Print and shaded views of the part. All mm, measured from the part's lowest x, y and z. Coordinates: 2 decimals unless noted, no trailing zeros. Order: outer loops, then holes, each group sorted by start corner. A loop starts at its lowest first (then second) coordinate and runs counter-clockwise, first axis right, second up. Notation, with made-up numbers: (-38, 75.25) -> (-1, 75.25) arc R21 cw to (-1, 89.25) -> close; hole circle Ø3 at (31, -3). An arc over 180 degrees is marked (long way). Return JSON: item names as keys, results as strings. Group by question number.
1) Cut at A-A (z = 43). Write the cut outline in (x, y), and give its area (3 significant figures).
2) Flat gauge pins, fed straight in: pin 1 (4.5 mm diameter, centred on x = 96.5, y = 6.5, fed in from -Z); pin 2 (4.5 mm diameter, centred on x = 80, y = 6, fed in from +Z); pin 3 (1 mm diameter, centred on y = 4, z = 59.5, fed in from +X). Where does each tip first touch, or does it go through?
3) Cut at C-C (z = 27.5). Write the cut outline in (x, y), and give its area (3 significant figures).
4) Cut at B-B (x = 50). Write the cut outline in (y, z), and give its area (3 significant figures).
5) Probe line 1 (X direction, y = 3.25, z = 58.5); line 2 (X direction, y = 3.5, z = 27.5); line 3 (Z direction, x = 65.5, y = 6). List the from-to ranges inside material, lowest first.
6) Cut at D-D (y = 6). State how many separate pieces and enclosed holes the cut face has, and give its area (3 significant figures).
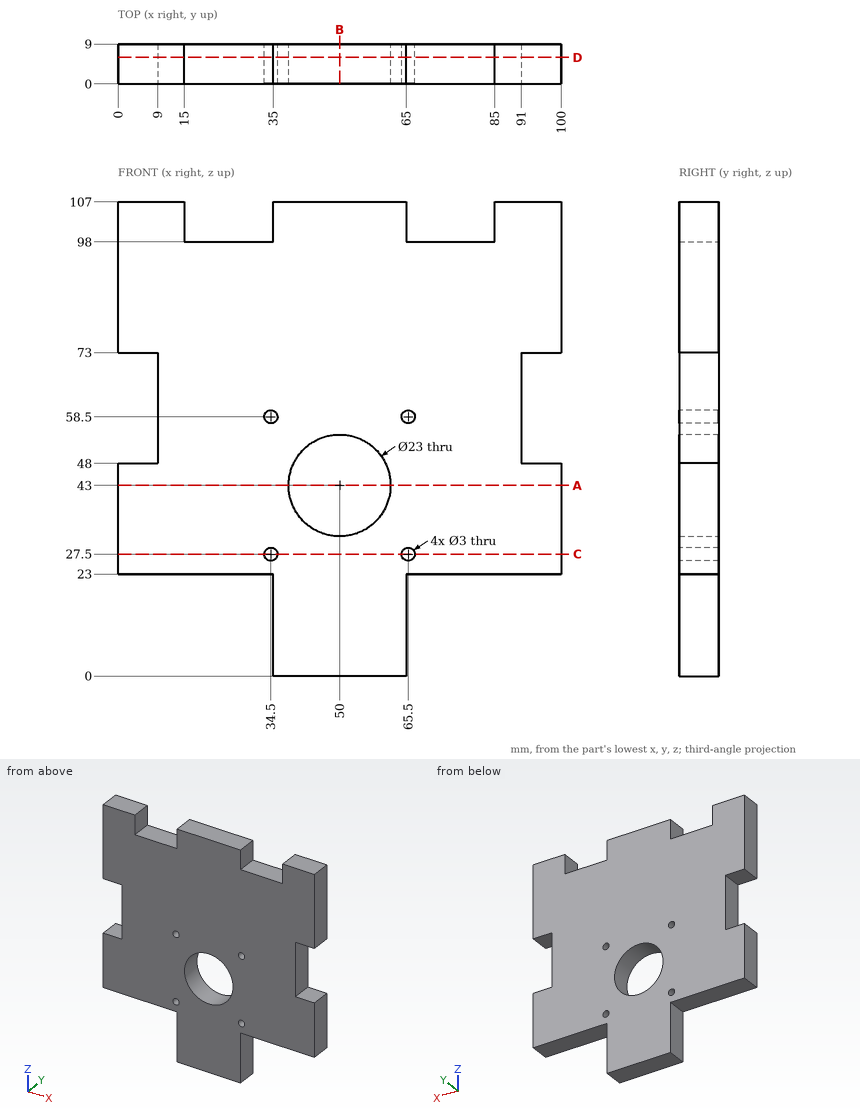
Answers below:
{
 "1": {"outline": "(0, 0) -> (38.5, 0) -> (38.5, 9) -> (0, 9) -> close; (61.5, 0) -> (100, 0) -> (100, 9) -> (61.5, 9) -> close", "area": "693 mm^2"},
 "2": {"pin 1": "stops at z = 23", "pin 2": "stops at z = 98", "pin 3": "stops at x = 91"},
 "3": {"outline": "(0, 0) -> (33, 0) -> (33, 9) -> (0, 9) -> close; (36, 0) -> (64, 0) -> (64, 9) -> (36, 9) -> close; (67, 0) -> (100, 0) -> (100, 9) -> (67, 9) -> close", "area": "846 mm^2"},
 "4": {"outline": "(0, 0) -> (9, 0) -> (9, 31.5) -> (0, 31.5) -> close; (0, 54.5) -> (9, 54.5) -> (9, 107) -> (0, 107) -> close", "area": "756 mm^2"},
 "5": {"line 1": "x = 9 to 33, 36 to 64, 67 to 91", "line 2": "x = 0 to 33, 36 to 64, 67 to 100", "line 3": "z = 23 to 26, 29 to 57, 60 to 98"},
 "6": {"separate pieces": "1", "enclosed holes": "5", "area": "7,840 mm^2"}
}
